Geometry: final body of the model. Coordinates: model frame, mm. Give positions to 0.01 mm unless a question says otherwise; leave off trailing zeros. Order: outer loops, then holes, each group sorted by start corner. A loop starts at its lowest first (then second) coordinate and runs counter-clockwise, first axis right, second up. Notation, with made-up numbers: (15, -4) -> (68, -4) arc R6 ccw to (68, 7) -> close; hole circle Ø11 at (74.5, -13). An arc over 180 degrees is marked (long way). Answer in a Markdown table with one row per item. Add a question column.
Q1. Cut plane B-B on y = -2.25. Return the cut outline in (x, z), and give its area (3 significant figures).
Q2. Line query: line 1 along X through (y, z) = (-1.75, 99.5); line 2 along X through (y, z) = (-4.75, -203); line 3 along Y through (x, z) = (5.5, -68). Output: solid intervals per line, ascending. Write a range as from..to.
Q3. Cut plane A-A on z = 1.5. Return the cut outline in (x, y), and give its area (3 significant figures).
Q4. Contact query for flat-ended pins moving along their axis: P1, Ø1, axis at y = 3.5, z = -17.5, coming from the -X side; P2, Ø2, axis at y = 3, z = -46.5, coming from the -X side; P3, Ø2, axis at y = 0.5, z = 178.5, coming from the -X side; P4, Ø1, axis at x = -5.5, y = -4.5, coming from the +Z side. Output: stop coordinate, or through.
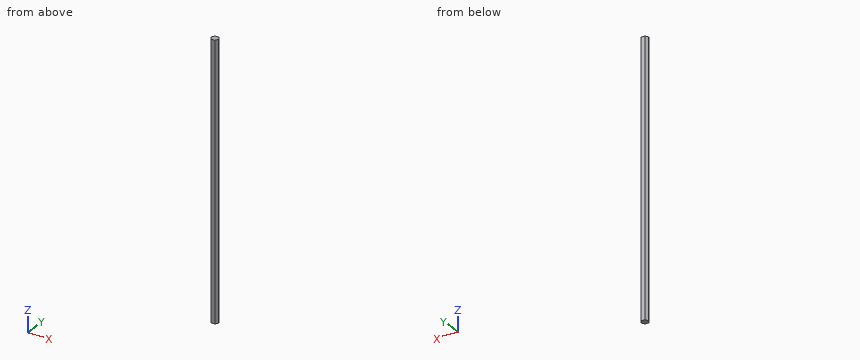
Autodesk Inventor part; units mm, degrees
ref_plane "YZ Plane" through (0, 0, 0) normal (1, 0, 0) x (0, 1, 0)
ref_plane "XZ Plane" through (0, 0, 0) normal (0, 1, 0) x (-1, 0, 0)
ref_plane "XY Plane" through (0, 0, 0) normal (0, 0, 1) x (1, 0, 0)
sketch "Sketch1" plane through (0, 0, 0) normal (0, 0, 1) x (1, 0, 0)
  line L0 (-3.6719, 6.36) -> (3.6719, 6.36)
  line L1 (3.6719, 6.36) -> (7.3439, 0)
  line L2 (7.3439, 0) -> (3.6719, -6.36)
  line L3 (3.6719, -6.36) -> (-3.6719, -6.36)
  line L4 (-3.6719, -6.36) -> (-7.3439, 0)
  line L5 (-7.3439, 0) -> (-3.6719, 6.36)
  point P0 (0, 0)
  point P1 (0, 0)
  dimension "d0" = 7.3439
extrude "Extrusion1" add sketch "Sketch1" along normal mid plane 533.4
properties part number "Hex_shaft"
Completed:
| question | item | result |
|---|---|---|
| 1 | outline | (-6.04, -266.7) -> (6.04, -266.7) -> (6.04, 266.7) -> (-6.04, 266.7) -> close |
| 1 | area | 6,450 mm² |
| 2 | line 1 | x = -6.33..6.33 |
| 2 | line 2 | x = -4.6..4.6 |
| 2 | line 3 | y = -3.19..3.19 |
| 3 | outline | (-7.34, 0) -> (-3.67, -6.36) -> (3.67, -6.36) -> (7.34, 0) -> (3.67, 6.36) -> (-3.67, 6.36) -> close |
| 3 | area | 140 mm² |
| 4 | P1 | stops at x = -5.61 |
| 4 | P2 | stops at x = -6.19 |
| 4 | P3 | stops at x = -7.34 |
| 4 | P4 | passes through |
